Geometry: final body of the model. Coordinates: model frame, mm. Face numbers are marked on the shaded views. A direction names the side the tool comes from. Coordinates: 2 decimals unless noted, no trailing zeros. Order: outer loops, then holes, each group sorted by start corner. A loop starts at its lowest first (then second) coordinate and runs counter-clockwise, first axis right, second up. Notation, with made-up numbers: (6, 75) -> (45, 75) arc R37 cw to (45, 112) -> close; hole circle Ø11 at (39.5, 63.25). An arc over 180 degrees is marked (long way). Answer in a Markdown table with one row per item. Add a question column.
1) Section query B-B on z = 30. Return the cut outline in (x, y), then the cut area to 3 significant figures.
2) Section query C-C on z = 0. Return the cut outline in (x, y).
3) Section query A-A on x = 10. Return the cut outline in (y, z).
4) Contact query for flat-ended pins moving along their axis: P1, Ø8, axis at x = -50.67, z = 30, coming from the +Y side; P2, Ø4, axis at y = 5, z = 28, coming from the -X side; P3, Ø15, axis at x = -54, z = -15, coming from the -Y side; P4, Ø3, axis at x = 5.5, z = -39, coming from the +Y side. Output: stop coordinate, or through.
5) Set-up query: the marked faces 1, 2 and 3. Return all of +Z, -Z, +X, -X, +Y, -Y with unobstructed straight access to the full face (end or side cutting, diameter ignored); none if empty.
6) Ray query, line 1 (X direction, y = 33, z = 23); line 2 (Y direction, x = -24, z = 5); line 3 (Y direction, x = -47.5, z = -5). Return the intervals inside material, ascending. Write a range as from..to.
7) Section query D-D on y = 14. Return the cut outline in (x, z).
```python
from build123d import *

# Parameters (mm, degrees)
SKETCH5_W               = 120
SKETCH5_H               = 100
BASE_FLANGE1_DEPTH      = 0.7366
JOG1_START              = -50
JOG1_DEPTH              = 100
JOG1_2_DEPTH            = 100
SKETCH15_R              = 12
CUT_EXTRUDE1_DEPTH      = 2
SKETCH21_R              = 5
CUT_EXTRUDE3_DEPTH      = 1.8
CUT_EXTRUDE4_DEPTH      = 2
CUT_EXTRUDE4_DEPTH_BACK = 1.8
SKETCH22_R              = 7.5


# Read off the part's stored shape, not the designer's step: Jog1
# Sheet-metal steps are written as plain solids
with BuildPart() as part:
    # Sketch5 → Base-Flange1 (new body)
    with BuildSketch(Plane(origin=(0, 0, 0), x_dir=(1, 0, 0), z_dir=(0, 1, 0))):
        Rectangle(SKETCH5_W, SKETCH5_H)
    extrude(amount=-BASE_FLANGE1_DEPTH)

    # Jog1 outline → Jog1 (cut)
    with BuildSketch(Plane.XY.offset(JOG1_START)):
        with BuildLine():
            ThreePointArc((-39.132213569, -0.7366), (-39.868813569, -0.539228625), (-40.408042194, 0))
            Line((-40.408042194, 0), (-60, 0))
            Line((-60, 0), (-60, -0.7366))
            Line((-60, -0.7366), (-39.132213569, -0.7366))
        make_face()
    extrude(amount=JOG1_DEPTH, mode=Mode.SUBTRACT)

    # Jog1 2 outline → Jog1 2 (add)
    with BuildSketch(Plane.XY.offset(JOG1_START)):
        with BuildLine():
            Line((-40.605413569, 38.5268), (-40.605413569, 0.7366))
            ThreePointArc((-40.605413569, 0.7366), (-40.555215496, 0.355307783), (-40.408042194, 0))
            Line((-40.408042194, 0), (-39.132213569, 0))
            ThreePointArc((-39.132213569, 0), (-39.653068424, 0.215745145), (-39.868813569, 0.7366))
            Line((-39.868813569, 0.7366), (-39.868813569, 38.5268))
            ThreePointArc((-39.868813569, 38.5268), (-40.300303859, 39.56850971), (-41.342013569, 40))
            Line((-41.342013569, 40), (-60, 40))
            Line((-60, 40), (-60, 39.2634))
            Line((-60, 39.2634), (-41.342013569, 39.2634))
            ThreePointArc((-41.342013569, 39.2634), (-40.821158714, 39.047654855), (-40.605413569, 38.5268))
        make_face()
    extrude(amount=JOG1_2_DEPTH)

    # Sketch15 → Cut-Extrude1 (cut)
    with BuildSketch(Plane(origin=(0, 0, 0), x_dir=(1, 0, 0), z_dir=(0, 1, 0))):
        with Locations(Location((10, 0, 0), (0, 0, 270))):
            Circle(SKETCH15_R)
    extrude(amount=-CUT_EXTRUDE1_DEPTH, mode=Mode.SUBTRACT)

    # Sketch21 → Cut-Extrude3 (cut)
    with BuildSketch(Plane(origin=(0, 40, 0), x_dir=(1, 0, 0), z_dir=(0, 1, 0))):
        with Locations(Location((-50.671006785, 30, 0), (0, 0, 270))):
            Circle(SKETCH21_R)
        with Locations(Location((-50.671006785, -30, 0), (0, 0, 270))):
            Circle(SKETCH21_R)
    extrude(amount=-CUT_EXTRUDE3_DEPTH, mode=Mode.SUBTRACT)

    # Sketch22 → Cut-Extrude4 (cut, two sides: drawn at the far end of the back side and taken through both)
    with BuildSketch(Plane(origin=(-40, 0, 0), x_dir=(0, 0, -1), z_dir=(1, 0, 0)).offset(-CUT_EXTRUDE4_DEPTH_BACK)):
        with Locations(Location((30, 19.6317, 0), (0, 0, 90))):
            Circle(SKETCH22_R)
        with Locations(Location((-30, 19.6317, 0), (0, 0, 90))):
            Circle(SKETCH22_R)
    extrude(amount=CUT_EXTRUDE4_DEPTH + CUT_EXTRUDE4_DEPTH_BACK, mode=Mode.SUBTRACT)


solid = part.part
```
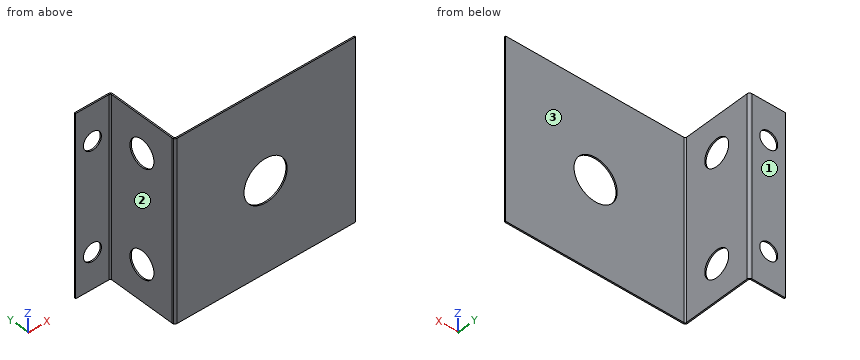
Result:
| question | item | result |
|---|---|---|
| 1 | outline | (-60, 39.26) -> (-55.67, 39.26) -> (-55.67, 40) -> (-60, 40) -> close; (-45.67, 39.26) -> (-41.34, 39.26) arc R0.74 cw to (-40.61, 38.53) -> (-40.61, 27.13) -> (-39.87, 27.13) -> (-39.87, 38.53) arc R1.47 ccw to (-41.34, 40) -> (-45.67, 40) -> close; (-40.61, 0.74) arc R1.47 ccw to (-39.13, -0.74) -> (60, -0.74) -> (60, 0) -> (-39.13, 0) arc R0.74 cw to (-39.87, 0.74) -> (-39.87, 12.13) -> (-40.61, 12.13) -> close |
| 1 | area | 98.7 mm2 |
| 2 | outline | (-60, 39.26) -> (-41.34, 39.26) arc R0.74 cw to (-40.61, 38.53) -> (-40.61, 0.74) arc R1.47 ccw to (-39.13, -0.74) -> (-2, -0.74) -> (-2, 0) -> (-39.13, 0) arc R0.74 cw to (-39.87, 0.74) -> (-39.87, 38.53) arc R1.47 ccw to (-41.34, 40) -> (-60, 40) -> close; (22, -0.74) -> (60, -0.74) -> (60, 0) -> (22, 0) -> close |
| 3 | outline | (-0.74, -50) -> (0, -50) -> (0, -12) -> (-0.74, -12) -> close; (-0.74, 12) -> (0, 12) -> (0, 50) -> (-0.74, 50) -> close |
| 4 | P1 | through |
| 4 | P2 | x = -40.61 |
| 4 | P3 | y = 39.26 |
| 4 | P4 | y = 0 |
| 5 | face 1 | +Z, -Z, +X, -X, +Y |
| 5 | face 2 | +Z, -Z, -X, -Y |
| 5 | face 3 | +Z, -Z, +X, +Y |
| 6 | line 1 | -40.61..-39.87 |
| 6 | line 2 | -0.74..0 |
| 6 | line 3 | 39.26..40 |
| 7 | outline | (-40.61, -50) -> (-39.87, -50) -> (-39.87, -34.95) -> (-40.61, -34.95) -> close; (-40.61, -25.05) -> (-39.87, -25.05) -> (-39.87, 25.05) -> (-40.61, 25.05) -> close; (-40.61, 34.95) -> (-39.87, 34.95) -> (-39.87, 50) -> (-40.61, 50) -> close |
